Model file for the job. Use its own axes, mm. A direction names the side the tool comes from. Give positions to 0.01 mm unless a question says otherwise; leave off trailing zeros. Order: outer loops, then holes, each group sorted by start corner. A loop starts at its lowest first (then second) coordinate and runs counter-clockwise, first axis right, second up. Notation, with made-up numbers: (70, 87) - (107, 87) arc R12 ccw to (107, 104) - close; hole circle Ø8 at (-22.5, 3). An arc over 180 degrees is marked (long way). Use CSV: the item, a comma, the result in double quotes. Start each with the question number.
(1) Band-saw the part on A-A, the plane y = 11.5. Give the cut face in (x, z).
(2) Pull direction Y, two halves, no side cores. Call faces 1 (the flat face through (2.31, 10.96, -5.42)), 2 (the flat face through (2, 7, 22.041)), 3 (the conical face through (27.6, 6.31, -11.92)): +Y half, -Y half, draft (parallel to the pull), parting line (faces both ways), or undercut.
(3) Band-saw the part on B-B, the plane x = -4. Give the cut face in (y, z).
(4) Drop flat-ended pins along their axis: pin 1 Ø3.5 at (x, z) = (17.8, 15.54) entering from +Y; pin 2 Ø2.5 at (x, y) = (-22.2, 6) entering from -Z. Give the stop position or say it passes through.
(5) Band-saw the part on D-D, the plane z = -0.5. Give the cut face in (x, y), then the cut area to 3 significant figures.
(6) Probe L1, parallel to Z at x = -11.5, y = 12.5; L2, parallel to X at y = 5.75, z = -24.5; L3, parallel to X at y = 5.5, z = -21.5. List the from-to ranges inside material, lowest first.
(7) Tool access for faces 4 (the cylindrical face through (-23.75, 7.42, 14.65)), 5 (the cylindrical face through (25.7, 6.1, -20.4)), 6 (the cylindrical face through (2.583, 4.056, -23.095)): list every direction of +Z, -Z, +X, -X, +Y, -Y with a clear straight run to the whole face (end or side of a thin tool).
(8) Band-saw the part on C-C, the plane y = 2.5. Give the cut face in (x, z).
from build123d import *

# Parameters (mm, degrees)
SKETCH1_W             = 70
SKETCH1_H             = 50
BOSS_EXTRUDE1_DEPTH   = 13.5
CUT_EXTRUDE1_DEPTH    = 78.5
SKETCH6_R             = 3
CUT_EXTRUDE2_DEPTH    = 200
M4_TAPPED_HOLE1_D     = 3.3
M4_TAPPED_HOLE1_DEPTH = 8
M4_TAPPED_HOLE1_TIP   = 0.991420021
M5_TAPPED_HOLE1_D     = 4.2
M5_TAPPED_HOLE1_DEPTH = 15
M5_TAPPED_HOLE1_TIP   = 1.2618073


# Read off the part's stored shape, not the designer's step: M5 Tapped Hole2
with BuildPart() as part:
    # Sketch1 → Boss-Extrude1 (new body)
    with BuildSketch(Plane(origin=(0, 0, 0), x_dir=(1, 0, 0), z_dir=(0, 1, 0))):
        with Locations((2.798036466, 2.959326788)):
            Rectangle(SKETCH1_W, SKETCH1_H)
    extrude(amount=BOSS_EXTRUDE1_DEPTH)

    # Sketch3 → Cut-Extrude1 (cut)
    with BuildSketch(Plane.ZY.offset(32.201963534)):
        Polygon((-2.959326788, 8.5), (-7.959326788, 13.5), (2.040673212, 13.5), align=None)
    extrude(amount=-CUT_EXTRUDE1_DEPTH, mode=Mode.SUBTRACT)

    # Sketch6 → Cut-Extrude2 (cut)
    with BuildSketch(Plane(origin=(0, 0, 0), x_dir=(1, 0, 0), z_dir=(0, 1, 0))):
        with Locations(Location((-12.201963534, -15.540673212, 0), (0, 0, 270))):
            Circle(SKETCH6_R)
        with Locations(Location((17.798036466, -15.540673212, 0), (0, 0, 270))):
            Circle(SKETCH6_R)
        with Locations(Location((-12.201963534, 21.459326788, 0), (0, 0, 270))):
            Circle(SKETCH6_R)
        with Locations(Location((17.798036466, 21.459326788, 0), (0, 0, 270))):
            Circle(SKETCH6_R)
    extrude(amount=CUT_EXTRUDE2_DEPTH, mode=Mode.SUBTRACT)

    # M4 Tapped Hole1
    with Locations(Plane(origin=(0, 0, 0), x_dir=(-1, 0, 0), z_dir=(0, -1, 0))):
        with Locations((-2.798036466, -15.540673212), (-2.798036466, 21.459326788)):
            Hole(M4_TAPPED_HOLE1_D / 2, depth=M4_TAPPED_HOLE1_DEPTH)
            with Locations((0, 0, -(M4_TAPPED_HOLE1_DEPTH + M4_TAPPED_HOLE1_TIP / 2))):  # 118° drill point
                Cone(0, M4_TAPPED_HOLE1_D / 2, M4_TAPPED_HOLE1_TIP, mode=Mode.SUBTRACT)

    # M5 Tapped Hole1
    with Locations(Plane(origin=(0, 0, -27.959326788), x_dir=(-1, 0, 0), z_dir=(0, 0, -1))):
        with Locations((-27.798036466, 6), (22.201963534, 6)):
            Hole(M5_TAPPED_HOLE1_D / 2, depth=M5_TAPPED_HOLE1_DEPTH)
            with Locations((0, 0, -(M5_TAPPED_HOLE1_DEPTH + M5_TAPPED_HOLE1_TIP / 2))):  # 118° drill point
                Cone(0, M5_TAPPED_HOLE1_D / 2, M5_TAPPED_HOLE1_TIP, mode=Mode.SUBTRACT)

    # M5 Tapped Hole2 outline → M5 Tapped Hole2 (revolve, cut)
    with BuildSketch(Plane(origin=(-22.201963534, 6, 0), x_dir=(1, 0, 0), z_dir=(0, -1, 0))):
        Polygon((0, 5.778865912), (2.1, 7.040673212), (2.1, 22.040673212), (0, 22.040673212), align=None)
    revolve(axis=Axis((-22.201963534, 6, 0), (0, 0, 1)), mode=Mode.SUBTRACT)

    # M5 Tapped Hole2 2 outline → M5 Tapped Hole2 2 (revolve, cut)
    with BuildSketch(Plane(origin=(27.798036466, 6, 0), x_dir=(1, 0, 0), z_dir=(0, -1, 0))):
        Polygon((0, 5.778865912), (2.1, 7.040673212), (2.1, 22.040673212), (0, 22.040673212), align=None)
    revolve(axis=Axis((27.798036466, 6, 0), (0, 0, 1)), mode=Mode.SUBTRACT)


solid = part.part
Answer block:
1,outline,"(-32.2, -27.96) - (37.8, -27.96) - (37.8, -5.96) - (-32.2, -5.96) - close; (-32.2, 0.04) - (37.8, 0.04) - (37.8, 22.04) - (-32.2, 22.04) - close; hole circle Ø6 at (-12.2, -21.46); hole circle Ø6 at (-12.2, 15.54); hole circle Ø6 at (17.8, -21.46); hole circle Ø6 at (17.8, 15.54)"
2,face 1,"+Y half"
2,face 2,"draft"
2,face 3,"undercut"
3,outline,"(0, -27.96) - (13.5, -27.96) - (13.5, -7.96) - (8.5, -2.96) - (13.5, 2.04) - (13.5, 22.04) - (0, 22.04) - close"
4,pin 1,"passes through"
4,pin 2,"stops at z = -12.45"
5,outline,"(-32.2, 0) - (37.8, 0) - (37.8, 10.96) - (-32.2, 10.96) - close"
5,area,"767 mm2"
6,L1,"z = -27.96 to -24.38, -18.54 to -6.96, 1.04 to 12.62, 18.46 to 22.04"
6,L2,"x = -32.2 to -24.29, -20.12 to 25.71, 29.88 to 37.8"
6,L3,"x = -32.2 to -24.24, -20.16 to -15.2, -9.2 to 1.15, 4.45 to 14.8, 20.8 to 25.76, 29.84 to 37.8"
7,face 4,"+Z"
7,face 5,"-Z"
7,face 6,"-Y"
8,outline,"(-32.2, -27.96) - (37.8, -27.96) - (37.8, 22.04) - (-32.2, 22.04) - close; hole circle Ø6 at (-12.2, -21.46); hole circle Ø6 at (-12.2, 15.54); hole circle Ø3.3 at (2.8, -21.46); hole circle Ø3.3 at (2.8, 15.54); hole circle Ø6 at (17.8, -21.46); hole circle Ø6 at (17.8, 15.54)"
